Build history of the part. All positions in model axes, mm. Face numbers are marked on the shaded views. Give positions to 0.01 mm unless a question says otherwise; leave off trailing zeros. Loops run counter-clockwise (first coordinate to the right, second up) from the corner with the lowest first, then second, coordinate; pieces in that order, holes last. Notation, with made-up numbers: (38.5, -27.5) -> (47.5, -27.5) arc R25 cw to (47.5, -2.5) -> close; hole circle Ø3 at (-3.75, 54). An arc over 180 degrees is marked (long way). Answer as a JSON object with one key per item and string values. Group by question number.
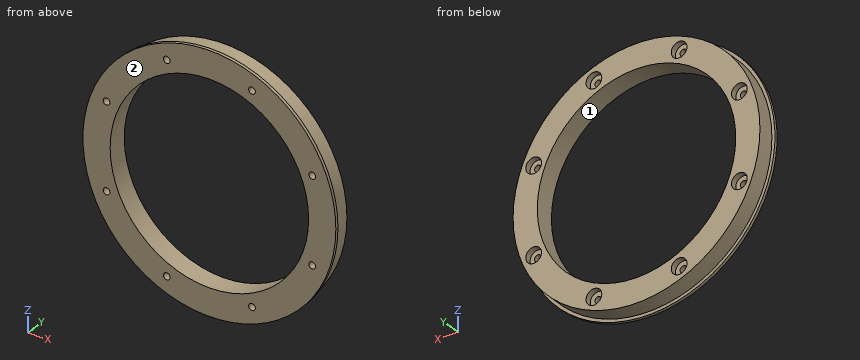
Autodesk Inventor part; units mm, degrees
ref_plane "YZ Plane" through (0, 0, 0) normal (1, 0, 0) x (0, 1, 0)
ref_plane "XZ Plane" through (0, 0, 0) normal (0, 1, 0) x (-1, 0, 0)
ref_plane "XY Plane" through (0, 0, 0) normal (0, 0, 1) x (1, 0, 0)
sketch "Sketch5" plane through (0, 0, 0) normal (0, 0, 1) x (1, 0, 0)
  line L0 (0, 0) -> (0, 33)
  line L1 (164, 0) -> (164, 33)
  line L2 (164, 33) -> (204, 33)
  line L3 (204, 33) -> (204, 5)
  line L4 (204, 5) -> (209, 5)
  line L5 (209, 5) -> (209, 0)
  line L6 (209, 0) -> (164, 0)
  point P0 (186.5, 0)
  dimension "d16" = 328
  dimension "d17" = 408
  dimension "d19" = 28
  dimension "d20" = 5
  dimension "d21" = 5
revolve "Revolution1" add sketch "Sketch5" angle 360 about axis through (0, 0, 0) along (0, 1, 0)
sketch "Sketch6" plane through (0, 33, 0) normal (0, 1, 0) x (1, 0, 0)
  circle A0 centre (0, 0) radius 184
  line L0 (0, 0) -> (-70.4138, 169.9938)
  line L1 (0, 0) -> (0, 184)
  dimension "d23" = 368
  dimension "d34" = 22.5
hole "Hole1" at (-70.4138, 33, -169.9938) direction (0, -1, 0) diameter 11 end through all counterbore diameter 26 counterbore depth 10
pattern_circular "Circular Pattern2" count 8 over 360 about axis through (0, -10, 0) along (0, 1, 0) of "Hole1"
equation "\"d29\" = Thickness"
properties part number "DMF 01 32 Барабан Опорное кольцо КОРМА v2.1"
(1) Saw through at A-A on x = 0. List the corners of the cut face in (y, z).
(2) Pull direction Z, two halves, no side cores. Call the marked faces 1 and 2: pulls with the +Z half, pulls with the -Z half, needs draft (parallel to the pull), parting line crosses it, or undercut.
(3) Probe line 1 along X through (y, z) = (7.5, 0); line 2 along Z through (x, y) = (-177, 31); line 3 along X through (y, z) = (16.5, -74). List the from-to ranges inside material, lowest first. Write a range as [from, to].
(4) Saw through at B-B on z = 0. List the corners of the cut face in (x, y).
(5) Pin check, flat tips, straight feed: pin 1 (15.5 mm diameter, centred on x = 169.99, z = -70.41, fed in from +Y); pin 2 (14.5 mm diameter, centred on x = -70.41, z = -169.99, fed in from -Y); pin 3 (6 mm diameter, centred on y = 23, z = -23, fed in from -X); pin 4 (4 mm diameter, centred on y = 19, z = -21.5, fed in from +X). Stop position of each tip, or through.
Calculated:
{
 "1": {"outline": "(0, -209) -> (5, -209) -> (5, -204) -> (33, -204) -> (33, -164) -> (0, -164) -> close; (0, 164) -> (33, 164) -> (33, 204) -> (5, 204) -> (5, 209) -> (0, 209) -> close"},
 "2": {"face 1": "undercut", "face 2": "needs draft"},
 "3": {"line 1": "x = [-204, -164], [164, 204]", "line 2": "z = [-101.42, -81.36], [-59.46, 59.46], [81.36, 101.42]", "line 3": "x = [-190.11, -174.16], [-165.82, -146.36], [146.36, 165.82], [174.16, 190.11]"},
 "4": {"outline": "(-209, 0) -> (-164, 0) -> (-164, 33) -> (-204, 33) -> (-204, 5) -> (-209, 5) -> close; (164, 0) -> (209, 0) -> (209, 5) -> (204, 5) -> (204, 33) -> (164, 33) -> close"},
 "5": {"pin 1": "stops at y = 23", "pin 2": "stops at y = 0", "pin 3": "stops at x = -203.02", "pin 4": "stops at x = 203.07"}
}
